Check sheet for the modelled part. Datum: model origin and axes. Units: mm. A direction names the side the tool comes from. Round coordinates to 2 decimals unless told otherwise and drop trailing zeros. Loops run counter-clockwise (first coordinate to the right, second up) from the corner with the lowest first, then second, coordinate; pieces in that order, holes last. Notation, with made-up numbers: (79, -28.5) -> (91, -28.5) arc R23 ccw to (91, -17.5) -> close; hole circle Ø5 at (-21.75, -10.75). An arc over 180 degrees is marked (long way). One line per item, written item: value. Start each with the question number.
1. Go/stop test with flat-tipped pins: pin 1 (10 mm diameter, centred on x = -8.5, z = 58.5, fed in from -Y); pin 2 (1 mm diameter, centred on x = 4, z = 62.5, fed in from +Y); pin 3 (10 mm diameter, centred on y = -6.5, z = 58, fed in from -X). Record where each tip stops, or that it passes through.
2. Cross-section at A-A on z = 41.5. Record the cut outline in (x, y).
3. Set-up check for faces 1 (the face through (-2.415, 18.392, 82.421)), 2 (the face through (-15, -1, 30)): record each of +Z, -Z, +X, -X, +Y, -Y from which the full face is reachable in a straight line by a thin tool's end or side.
4. Release check for a two-part mould opening along X. For faces 3 (the face through (-2.415, 18.392, 48.523)), 4 (the face through (-15, -15, 89.45)), 5 (the face through (-2.764, -12.447, 51.449)), 6 (the face through (12.507, 3.939, 71.813)) record: +X half, -X half, draft (parallel to the pull), parting line (faces both ways), or undercut.
5. Material ranges on L1, parallel to X at y = 0.5, z = 61; L2, parallel to Y at x = 0, z = 43; L3, parallel to Y at x = 0, z = 84.75, recorded low to high.
from build123d import *

# Parameters (mm, degrees)
FILLET_R    = 6
FILLET002_R = 2


with BuildPart() as part:
    # Sketch003 → Revolution002 (revolve)
    with BuildSketch(Plane.XZ):
        Polygon((12.75, 30), (12.75, 68), (12.75, 71.45), (18.55, 77.25), (18.55, 89.45), (40, 89.45), (18.55, 68), (18.55, 30), align=None)
    revolve(axis=Axis((0, 0, 0), (0, 0, 1)))

    # Fillet
    fillet_edges = [part.edges().sort_by_distance(p)[0] for p in [
        (-18.55, 0, 68),
    ]]
    fillet(fillet_edges, radius=FILLET_R)

    # Fillet002
    fillet002_edges = [part.edges().sort_by_distance(p)[0] for p in [
        (-18.55, 0, 89.45),
        (-40, 0, 89.45),
        (-12.75, 0, 30),
        (-18.55, 0, 30),
    ]]
    fillet(fillet002_edges, radius=FILLET002_R)


solid = part.part
Taken from the geometry:
1. pin 1: stops at y = -18.22
1. pin 2: stops at y = 18.22
1. pin 3: stops at x = -18.49
2. outline: circle Ø37.1 at (0, 0); hole circle Ø25.5 at (0, 0)
3. face 1: +Z
3. face 2: -Z, +X, -X, +Y, -Y
4. face 3: parting line
4. face 4: draft
4. face 5: undercut
4. face 6: undercut
5. L1: x = -18.54 to -12.74, 12.74 to 18.54
5. L2: y = -18.55 to -12.75, 12.75 to 18.55
5. L3: y = -35.3 to -18.55, 18.55 to 35.3
